Part print with two shaded views. Sizes in mm from the minimum x, y, z corner. Give positions to 0.01 mm unless a question says otherwise; leave off trailing zeros. Write each loop counter-clockwise with the first axis right and the second up, starting at its lowest first coordinate (ties: lowest second). Pieces come first, ordered by that corner, then holes.
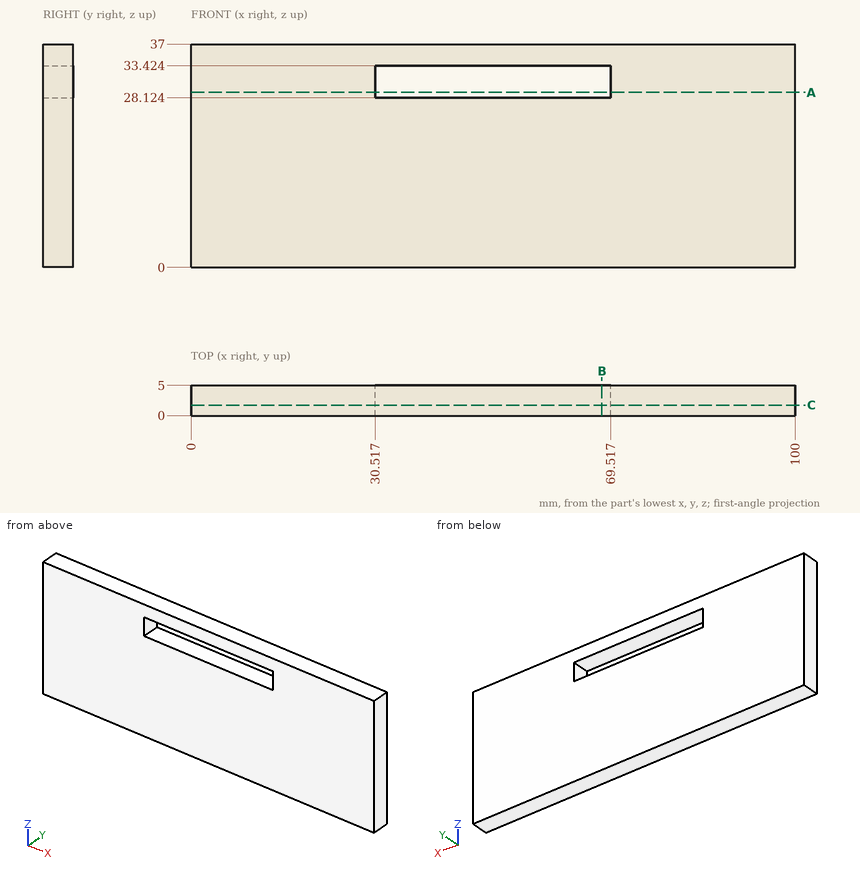
(1) Probe line 1 (X direction, y = 3.1, z = 32); line 2 (Z direction, x = 56, y = 0.85) (1 decimal). List the from-to ranges inside material, lowest first.
(2) Saw through at B-B, the plane x = 68. List the corners of the cut face in (y, z) (1 decimal).
(3) Saw through at C-C, the plane y = 1.75. List the corners of the cut face in (x, z) (1 decimal), plus the area to 3 significant figures.
(4) Saw through at A-A, the plane z = 29. List the corners of the cut face in (x, y), plus the area to 3 significant figures.
Computed values:
1. line 1: x = 0 to 30.52, 69.52 to 100
1. line 2: z = 0 to 28.1, 33.4 to 37
2. outline: (0, 0) - (5, 0) - (5, 28.1) - (0, 28.1) - close; (0, 33.4) - (5, 33.4) - (5, 37) - (0, 37) - close
3. outline: (0, 0) - (100, 0) - (100, 37) - (0, 37) - close; hole (30.5, 28.1) - (69.5, 28.1) - (69.5, 33.4) - (30.5, 33.4) - close
3. area: 3,490 mm2
4. outline: (0, 0) - (30.52, 0) - (30.52, 5) - (0, 5) - close; (69.52, 0) - (100, 0) - (100, 5) - (69.52, 5) - close
4. area: 305 mm2
